Work out the finished part from the listing and answer in its coordinate system (mm). Face numbers are marked on the shaded views. Give positions to 0.01 mm unless a question says otherwise; leave off trailing zeros. Write each loop counter-clockwise with the first axis right and the second up, starting at its lowest first coordinate (ties: lowest second). Pieces come first, ordered by that corner, then holes. Notation, with made-up numbers: (69.25, -29.75) - (114.25, -29.75) arc R17 cw to (114.25, 1.25) - close; hole circle Ø2 at (-3.75, -35). An arc over 180 degrees is marked (long way). Write each question's results on one line, items separated by ' | '. Start each with the question number.
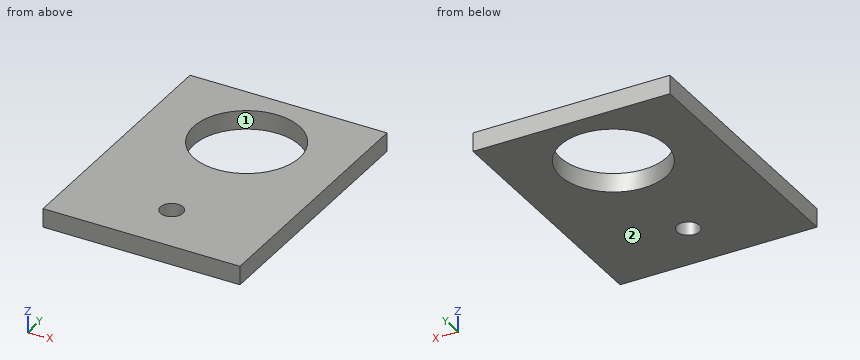
from build123d import *

# Parameters (mm, degrees)
F0_W     = 55.6
F0_H     = 43.07
F0_R     = 15
F0_H_2   = 30
F0_R_2   = 3.175
F1_DEPTH = 5.3


with BuildPart() as f1:
    # F0 (on Top) → F1 (new body)
    with BuildSketch(Plane.XY):
        Rectangle(F0_W, F0_H)
        with Locations((0, 0.7)):
            Circle(F0_R, mode=Mode.SUBTRACT)
        with Locations((0, -36.535)):
            Rectangle(F0_W, F0_H_2)
        with Locations((0, -36.535)):
            Circle(F0_R_2, mode=Mode.SUBTRACT)
    extrude(amount=F1_DEPTH)


solid = f1.part
Q1. A cutting plane is placed at D-D, the plane y = 13. Write down the section's boundary in (x, z).
Q2. Given pin 1 (5 mm diameter, centred on x = 0, y = -36.535, fed in from +Z), flat-ended and moving along its own axis, determine where the tip first touches the part or whether it passes through.
Q3. A cutting plane is placed at C-C, the plane z = 4.2. Write down the section's boundary in (x, y) (3 decimals).
Q4. Consider L1, parallel to Y at x = 0, z = 2.55 (3 decimals); L2, parallel to Y at x = -11.5, z = 2.5 (3 decimals); L3, parallel to Y at x = 6.5, z = 3.2 (1 decimal). Determine where each line is inside the solid, lowest interval first.
Q5. A cutting plane is placed at A-A, the plane x = 0. Write down the section's boundary in (y, z) (3 decimals), and give its area (3 significant figures).
Q6. The mould has two halves that part along X. Classify the marked faces 1 and 2: pulls with the +X half, pulls with the -X half, needs draft (parallel to the pull), parting line crosses it, or undercut.
Q7. A cutting plane is placed at B-B, the plane y = 0.7. Write down the section's boundary in (x, z), and give its area (3 significant figures).
Result:
1) outline: (-27.8, 0) - (-8.59, 0) - (-8.59, 5.3) - (-27.8, 5.3) - close; (8.59, 0) - (27.8, 0) - (27.8, 5.3) - (8.59, 5.3) - close
2) pin 1: passes through
3) outline: (-27.8, -51.535) - (27.8, -51.535) - (27.8, 21.535) - (-27.8, 21.535) - close; hole circle Ø30 at (0, 0.7); hole circle Ø6.35 at (0, -36.535)
4) L1: y = -51.535 to -39.71, -33.36 to -14.3, 15.7 to 21.535 | L2: y = -51.535 to -8.931, 10.331 to 21.535 | L3: y = -51.5 to -12.8, 14.2 to 21.5
5) outline: (-51.535, 0) - (-39.71, 0) - (-39.71, 5.3) - (-51.535, 5.3) - close; (-33.36, 0) - (-14.3, 0) - (-14.3, 5.3) - (-33.36, 5.3) - close; (15.7, 0) - (21.535, 0) - (21.535, 5.3) - (15.7, 5.3) - close | area: 195 mm2
6) face 1: undercut | face 2: needs draft
7) outline: (-27.8, 0) - (-15, 0) - (-15, 5.3) - (-27.8, 5.3) - close; (15, 0) - (27.8, 0) - (27.8, 5.3) - (15, 5.3) - close | area: 136 mm2
